Read the model definition and answer for the solid it produces. Units are mm, in the model's axes. A direction names the side the tool comes from. Coordinates: 2 decimals unless noted, no trailing zeros. Loops run counter-clockwise (first coordinate to the right, second up) from the corner with the lowest first, then second, coordinate; pieces in that order, holes last. Notation, with made-up numbers: M 11.25,13 L 49.25,13 A33 ccw 49.25,41 Z; hole C 11.5,11 d8. An arc over 180 degrees is marked long. Put each result on its own line as item: value.
from build123d import *

# Parameters (mm, degrees)
EXTRUDE_2_DEPTH              = 5
EXTRUDE_2_DEPTH_BACK         = 10
SKETCH_1_R                   = 5
SKETCH_2_R                   = 11
SKETCH_2_R_2                 = 1.5
EXTRUDE_3_DEPTH              = 3.5
HOLE_WIZARD_M8_1_D           = 6.8
HOLE_WIZARD_M8_1_DEPTH       = 22.25
HOLE_WIZARD_M8_1_CSINK_D     = 8.05
HOLE_WIZARD_M8_1_CSINK_ANGLE = 90
HOLE_WIZARD_M8_1_TIP         = 2.042926105


with BuildPart() as part:
    # 草图1 → 凸台-拉伸2 (new, two sides: drawn at the far end of the back side and taken through both)
    with BuildSketch(Plane(origin=(0, 0, 0), x_dir=(1, 0, 0), z_dir=(0, 1, 0)).offset(-EXTRUDE_2_DEPTH_BACK)):
        with Locations(Location((0, 0, 0), (0, 0, 270))):
            Circle(SKETCH_1_R)
    extrude(amount=EXTRUDE_2_DEPTH + EXTRUDE_2_DEPTH_BACK)

    # 草图2 → 凸台-拉伸3 (add)
    with BuildSketch(Plane(origin=(0, 0, 0), x_dir=(1, 0, 0), z_dir=(0, 1, 0))):
        with Locations(Location((0, 0, 0), (0, 0, 270))):
            Circle(SKETCH_2_R)
        with Locations(Location((8, 0, 0), (0, 0, 270))):
            Circle(SKETCH_2_R_2, mode=Mode.SUBTRACT)
        with Locations(Location((0, 8, 0), (0, 0, 270))):
            Circle(SKETCH_2_R_2, mode=Mode.SUBTRACT)
        with Locations(Location((-8, 0, 0), (0, 0, 270))):
            Circle(SKETCH_2_R_2, mode=Mode.SUBTRACT)
        with Locations(Location((0, -8, 0), (0, 0, 270))):
            Circle(SKETCH_2_R_2, mode=Mode.SUBTRACT)
    extrude(amount=EXTRUDE_3_DEPTH)

    # M8 螺纹孔1
    with Locations(Plane(origin=(0, 5, 0), x_dir=(1, 0, 0), z_dir=(0, 1, 0))):
        with Locations((0, 0)):
            CounterSinkHole(HOLE_WIZARD_M8_1_D / 2, HOLE_WIZARD_M8_1_CSINK_D / 2, depth=HOLE_WIZARD_M8_1_DEPTH, counter_sink_angle=HOLE_WIZARD_M8_1_CSINK_ANGLE)
            with Locations((0, 0, -(HOLE_WIZARD_M8_1_DEPTH + HOLE_WIZARD_M8_1_TIP / 2))):  # 118° drill point
                Cone(0, HOLE_WIZARD_M8_1_D / 2, HOLE_WIZARD_M8_1_TIP, mode=Mode.SUBTRACT)


solid = part.part
1) Find section B-B, the plane x = 8. Write down the section's boundary in (y, z), plus the area to 3 significant figures.
Answer list:
outline: M 0,-7.55 L 3.5,-7.55 L 3.5,-1.5 L 0,-1.5 Z; M 0,1.5 L 3.5,1.5 L 3.5,7.55 L 0,7.55 Z
area: 42.3 mm^2
2) Find section D-D, the plane y = -7.75. Write down the section's boundary in (x, z).
Answer list:
outline: C 0,0 d10; hole C 0,0 d6.8
3) Find section C-C, the plane z = -8.5. Write down the section's boundary in (x, y), plus the area to 3 significant figures.
Answer list:
outline: M -6.98,0 L -1.41,0 L -1.41,3.5 L -6.98,3.5 Z; M 1.41,0 L 6.98,0 L 6.98,3.5 L 1.41,3.5 Z
area: 39.0 mm^2
4) Given pin 1 Ø1.5 at (x, z) = (6, -2) entering from -Y; pin 2 Ø1 at (x, y) = (-2.5, -6.5) entering from -Z; pin 3 Ø5 at (x, y) = (6.5, -3) entering from -Z, each flat-ended and moving along its own axis, determine where each tip first touches the part or whether it passes through.
Answer list:
pin 1: stops at y = 0
pin 2: stops at z = -4.58
pin 3: stops at z = -3
5) Determine the mould class of faces 4 (the cylindrical face through (0.74, -2.91, 3.32)), 5 (the cylindrical face through (-4.88, 4.24, -1.08)), 6 (the flat face through (-5, 0, 2)) for opening direction X: released by +X, released by -X, zero draft, split by the parting line, or undercut.
Answer list:
face 4: undercut
face 5: split by the parting line
face 6: zero draft
6) Straight lines are drawn through the part: line 1 (Y direction, x = -6.75, z = 8); line 2 (Z direction, x = 0, y = -3.25); line 3 (X direction, y = 2.5, z = -9). For each, find the intervals that lie inside material, in ascending order. Write a range as [from, to].
Answer list:
line 1: y = [0, 3.5]
line 2: z = [-5, -3.4], [3.4, 5]
line 3: x = [-6.32, -1.12], [1.12, 6.32]
7) Find section A-A, the plane z = 0. Write down the section's boundary in (x, y) (3 decimals), plus the area to 3 significant figures.
Answer list:
outline: M -11,0 L -9.5,0 L -9.5,3.5 L -11,3.5 Z; M -6.5,0 L -5,0 L -5,-10 L -3.4,-10 L -3.4,4.375 L -4.025,5 L -5,5 L -5,3.5 L -6.5,3.5 Z; M 3.4,-10 L 5,-10 L 5,0 L 6.5,0 L 6.5,3.5 L 5,3.5 L 5,5 L 4.025,5 L 3.4,4.375 Z; M 9.5,0 L 11,0 L 11,3.5 L 9.5,3.5 Z
area: 68.6 mm^2
8) Which of the six approach directions +Z, -Z, +X, -X, +Y, -Y give full straight-line access (tool end or side, diameter ignored) to faces 1 (the cylindrical face through (-4.88, -5.07, -1.08)), 2 (the cylindrical face through (-9.464, 1.726, -0.325)), 3 (the flat face through (-5, 3.5, 2))?
Answer list:
face 1: -Y
face 2: +Y, -Y
face 3: +Y
